Could you check a few things on this model? Use its own coordinates, in mm. A direction names the side the tool comes from. Give positions to 0.01 mm unless a question says otherwise; leave off trailing zeros. Write each loop counter-clockwise with the first axis right and the second up, starting at its lowest first coordinate (ties: lowest second). Pieces come first, ordered by that corner, then holes. Notation, with made-up numbers: (54.5, 0.25) -> (95.5, 0.25) arc R4 cw to (95.5, 6.25) -> close; hole circle Ø10 at (46, 38). An arc over 180 degrees is marked (long way). Write item = value, one per line. Start each with the question number.
Autodesk Inventor part; units mm, degrees
ref_plane "YZ Plane" through (0, 0, 0) normal (1, 0, 0) x (0, 1, 0)
ref_plane "XZ Plane" through (0, 0, 0) normal (0, 1, 0) x (-1, 0, 0)
ref_plane "XY Plane" through (0, 0, 0) normal (0, 0, 1) x (1, 0, 0)
sketch "Sketch1" plane through (0, 0, 0) normal (0, 1, 0) x (-1, 0, 0)
  circle A0 centre (1.1561, 1.8072) radius 3
  line L0 (4.1561, 4.8072) -> (-1.8439, 4.8072)
  line L1 (-1.8439, 4.8072) -> (-1.8439, -1.1928)
  line L2 (-1.8439, -1.1928) -> (4.1561, -1.1928)
  line L3 (4.1561, -1.1928) -> (4.1561, 4.8072)
  point P0 (0, 0)
  dimension "d0" = 6
extrude "Extrusion1" add sketch "Sketch1" along normal blind 10
extrude "Extrusion2" add sketch "Sketch1" against normal blind 20 contours A0
sketch "Sketch2" plane through (-4.1561, 10, 4.8072) normal (0, 0, 1) x (1, 0, 0)
  line L0 (0, -10) -> (0, 0)
  line L1 (6, -10) -> (0, -10)
  line L2 (0, -10) -> (0, -7)
  line L3 (0, -7) -> (6, -7)
  line L4 (6, -7) -> (6, -10)
  line L5 (0, 0) -> (6, 0)
  line L6 (0, -30) -> (6, -30)
  line L7 (3, -10) -> (6, -10)
  point P0 (4.1561, -10)
  dimension "d5" = 3
  dimension "d6" = 6
  dimension "d7" = 30
  dimension "d13" = 0
extrude "Extrusion3" add sketch "Sketch2" along normal blind 7
sketch "Sketch3" plane through (-4.1561, 0, -1.1928) normal (-1, 0, 0) x (0, 0, 1)
  line L0 (6, 3) -> (13, 3)
  line L1 (13, 3) -> (13, 0)
  arc A0 (9.5, 3) -> (13, 1.5) centre (12.6357, 5.4834) ccw
  point P0 (1.1928, 0)
  dimension "d10" = 4
extrude "Extrusion4" [suppressed]
fillet "Fillet1" [suppressed]
fillet "Fillet2" [suppressed]
fillet "Fillet3" [suppressed]
sketch "Sketch4" plane through (1.8439, 0, -1.1928) normal (1, 0, 0) x (0, 0, -1)
  line L0 (-6, 3) -> (-13, 3)
  line L1 (-6, 3) -> (-13, 0.7757)
  line L2 (-13, 3) -> (-13, 0)
  line L3 (-13, 0.7757) -> (-13, 3)
  line L4 (-6, 3) -> (-13, 3)
  line L5 (-13, 3) -> (-6, 3)
  point P0 (-1.1928, 0)
extrude "Extrusion5" cut sketch "Sketch4" against normal blind 10
sketch "Sketch5" plane through (0, 0, 0) normal (0, -1, 0) x (1, 0, 0)
  line L0 (-4.1561, 4.8072) -> (1.8439, 4.8072)
  line L1 (-4.1561, 11.8072) -> (1.8439, 11.8072)
  line L2 (1.8439, 4.8072) -> (0.8439, 4.8072)
  line L3 (0.8439, 4.8072) -> (0.8439, 11.8072)
  line L4 (0.8439, 11.8072) -> (1.8439, 11.8072)
  line L5 (1.8439, 11.8072) -> (1.8439, 4.8072)
  line L6 (-3.1561, 4.8072) -> (-4.1561, 4.8072)
  line L7 (-4.1561, 4.8072) -> (-4.1561, 11.8072)
  line L8 (-4.1561, 11.8072) -> (-3.1561, 11.8072)
  line L9 (-3.1561, 11.8072) -> (-3.1561, 4.8072)
  line L10 (-3.1561, 10.3072) -> (0.8439, 10.3072)
  point P0 (0, 0)
  dimension "d19" = 6
  dimension "d20" = 1
  dimension "d21" = 1
  dimension "d28" = 1.5
extrude "Extrusion6" cut sketch "Sketch5" against normal blind 10 contours L3 L1 L5 L0
extrude "Extrusion7" cut sketch "Sketch5" against normal blind 10 contours L7 L1 L9 L0
extrude "Extrusion8" add sketch "Sketch1" against normal blind 5 contours L3 L2 A0 | A0 L0 L3 | A0 L1 L0 | L2 L1 A0
sketch "Sketch6" plane through (0.8439, 0, 11.8072) normal (1, 0, 0) x (0, 0, -1)
  point P0 (11.8072, 0)
sketch "Sketch7" plane through (0.8439, 0, 11.8072) normal (1, 0, 0) x (0, 0, -1)
  point P0 (11.8072, 0)
extrude "Extrusion9" add sketch "Sketch5" along normal blind 3 contours L9 L10 L3 L0
sketch "Sketch9" plane through (0.8439, 0, 11.8072) normal (1, 0, 0) x (0, 0, -1)
  line L0 (7, -3) -> (1.5, 0)
  line L1 (1.5, 0) -> (7, 0)
  line L2 (7, -3) -> (7, 3)
  line L3 (1.5, 0) -> (1.5, -3)
  line L4 (1.5, -3) -> (7, -3)
  point P0 (11.8072, 0)
extrude "Extrusion10" cut sketch "Sketch9" against normal blind 5 contours L4 L3 L0
sketch "Sketch10" plane through (0, -5, 0) normal (0, -1, 0) x (1, 0, 0)
  line L0 (2.8439, 5.8072) -> (-5.1561, 5.8072)
  line L1 (-5.1561, 5.8072) -> (-5.1561, -2.1928)
  line L2 (-5.1561, -2.1928) -> (2.8439, -2.1928)
  line L3 (2.8439, -2.1928) -> (2.8439, 5.8072)
  line L4 (1.8439, 1.8072) -> (1.8439, 4.8072)
  line L5 (-1.1561, -1.1928) -> (1.8439, -1.1928)
  line L6 (1.8439, 4.8072) -> (-1.1561, 4.8072)
  line L7 (-4.1561, 4.8072) -> (-4.1561, 1.8072)
  point P0 (0, 0)
  dimension "d33" = 1
  dimension "d34" = 1
  dimension "d35" = 1
  dimension "d36" = 1
extrude "Extrusion11" add sketch "Sketch10" against normal blind 1
sketch "Sketch11" plane through (-1.1561, -20, 1.8072) normal (0, -1, 0) x (1, 0, 0)
  circle A0 centre (0, 0) radius 3
  circle A1 centre (0, 0) radius 3
  point P0 (1.1561, -1.8072)
  dimension "d39" = 6
extrude "Extrusion12" add sketch "Sketch11" along normal blind 15
properties part number "pin"
(1) On a 3-axis mill with a long thin cutter (end or side, diameter ignored), from which of +Z, -Z, +X, -X, +Y, -Y can I reach the whole of each face in a straight line? I mean faces 1 (the flat face through (-1, 3, -1.193)), 2 (the flat face through (1, -5, 5)), 3 (the flat face through (-4.156, 3, 2)), 4 (the flat face through (-1.13, -1.52, 7.52)). Say none if no direction works.
(2) Imagine slicing it at C-C (y = -21.5). Please give me the cut outline in (x, z).
(3) I'm going to push flat-ended pins straight in: pin 1 (1 mm diameter, centred on y = -17.5, z = 0, fed in from +X); pin 2 (8 mm diameter, centred on y = -20.5, z = 6, fed in from +X); pin 3 (2 mm diameter, centred on x = -4, y = -8, fed in from -Z); pin 4 (1 mm diameter, centred on x = 2, z = 4.5, fed in from +Y). Where does each tip first touch, or does it pass through?
(4) If I drill on line 1 along Y through (x, z) = (-4.5, 5); line 2 along Z through (x, y) = (-4, -2); line 3 along X through (y, z) = (-16, 2), over which ranges is the centre line in solid material (lowest first)? Write a range as from..to.
(5) Imagine slicing it at B-B (z = 1). Please give me the cut outline in (x, y), then the cut area to 3 significant figures.
(6) Imagine slicing it at A-A (x = -3.75). Please give me the cut outline in (y, z), then the cut area to 3 significant figures.
(7) Imagine slicing it at D-D (x = -1). Please give me the cut outline in (y, z), then the cut area to 3 significant figures.
Answers below:
q1.face_1 = -Z, +X, -X, +Y
q1.face_2 = -Y
q1.face_3 = +Z, -Z, -X, +Y
q1.face_4 = +Z, +X, -X
q2.outline = circle Ø6 at (-1.16, 1.81)
q3.pin_1 = 1.54
q3.pin_2 = 1.84
q3.pin_3 = -0.56
q3.pin_4 = 10
q4.line_1 = -5..-4
q4.line_2 = -1.19..4.81
q4.line_3 = -4.15..1.84
q5.outline = (-5.16, -5) -> (-4.05, -5) -> (-4.05, -35) -> (1.73, -35) -> (1.73, -5) -> (2.84, -5) -> (2.84, -4) -> (1.84, -4) -> (1.84, 10) -> (-4.16, 10) -> (-4.16, -4) -> (-5.16, -4) -> close
q5.area = 265 mm^2
q6.outline = (-35, 0.3) -> (-5, 0.3) -> (-5, -2.19) -> (-4, -2.19) -> (-4, -1.19) -> (10, -1.19) -> (10, 4.81) -> (-4, 4.81) -> (-4, 5.81) -> (-5, 5.81) -> (-5, 3.31) -> (-35, 3.31) -> close
q6.area = 182 mm^2
q7.outline = (-35, -1.19) -> (-5, -1.19) -> (-5, -2.19) -> (-4, -2.19) -> (-4, -1.19) -> (10, -1.19) -> (10, 4.81) -> (3, 4.81) -> (0.78, 11.81) -> (0, 11.81) -> (0, 10.31) -> (-3, 4.81) -> (-4, 4.81) -> (-4, 5.81) -> (-5, 5.81) -> (-5, 4.8) -> (-35, 4.8) -> close
q7.area = 293 mm^2
